```python
from build123d import *

# Parameters (mm, degrees)
F1_DEPTH = 39.177313
F2_R     = 16.31925
F3_R     = 30.097367
F4_DEPTH = 30.095011
F6_DEPTH = 26.99797


with BuildPart() as f1:
    # F0 (on Top) → F1 (new body)
    with BuildSketch(Plane.XY):
        Polygon((55.259834, -64.92503), (28.596808, 80.318935), (-83.856642, -15.393905), align=None)
    extrude(amount=F1_DEPTH)

    # F2
    f2_edges = [f1.edges().sort_by_distance(p)[0] for p in [
        (41.928321, 7.696953, 39.177313),
        (-14.298404, -40.159468, 39.177313),
        (-27.629917, 32.462515, 39.177313),
    ]]
    fillet(f2_edges, radius=F2_R)

    # F3 (on face) → F4 (join)
    with BuildSketch(Plane(origin=(0, 0, 0), x_dir=(1, 0, 0), z_dir=(0, 0, -1))):
        Circle(F3_R)
    extrude(amount=-F4_DEPTH)

    # F5 (on Top) → F6 (join)
    with BuildSketch(Plane.XY):
        Polygon((16.23941, -30.575463), (32.093639, -12.983671), (32.930897, 10.683324), (18.359422, 29.351473), (-4.80263, 34.285742), (-25.717478, 23.177331), (-34.598832, 1.223989), (-27.291009, -21.302071), (-7.213418, -33.860655), align=None)
    extrude(amount=F6_DEPTH)


solid = f1.part
```
Check sheet for the modelled part. Datum: model origin and axes. Units: mm. Give positions to 0.01 mm unless a question says otherwise; leave off trailing zeros. Loops run counter-clockwise (first coordinate to the right, second up) from the corner with the lowest first, then second, coordinate; pieces in that order, holes last. Notation, with made-up numbers: (-20.5, -9) - (19.5, -9) arc R33 cw to (19.5, 20) - close; hole circle Ø1 at (87.25, -3). An arc over 180 degrees is marked (long way). One line per question, with ' | ' between items. Start each with the question number.
1. Cross-section at B-B, the plane z = 37.5. Enter the section's corners in (x, y), plus the area to 3 significant figures.
2. Material ranges on line 1 along Z through (x, y) = (-71.5, -15); line 2 along X through (y, z) = (51.5, 14.5); line 3 along Z through (x, y) = (-77, -14), recorded low to high. Write a range as [from, to].
3. Cross-section at A-A, the plane z = 7.5. Enter the section's corners in (x, y), plus the area to 3 significant figures.
4. Gauge pin test, flat ends, axial feed: pin 1 Ø3 at (x, y) = (36, -28.5) entering from +Z; pin 2 Ø5 at (y, z) = (-35, 11) entering from +X; pin 3 Ø5 at (y, z) = (43, 32.5) entering from +X. Record the tip position at first contact, or that the pin passes through.
Check result:
1) outline: (-65.93, -12.1) - (43.45, -51.05) - (22.48, 63.15) - close | area: 5,840 mm2
2) line 1: z = [0, 34.13] | line 2: x = [-5.26, 33.89] | line 3: z = [0, 32.81]
3) outline: (-83.86, -15.39) - (55.26, -64.93) - (28.6, 80.32) - close | area: 9,440 mm2
4) pin 1: stops at z = 38.99 | pin 2: stops at x = 50.23 | pin 3: stops at x = 33.86
